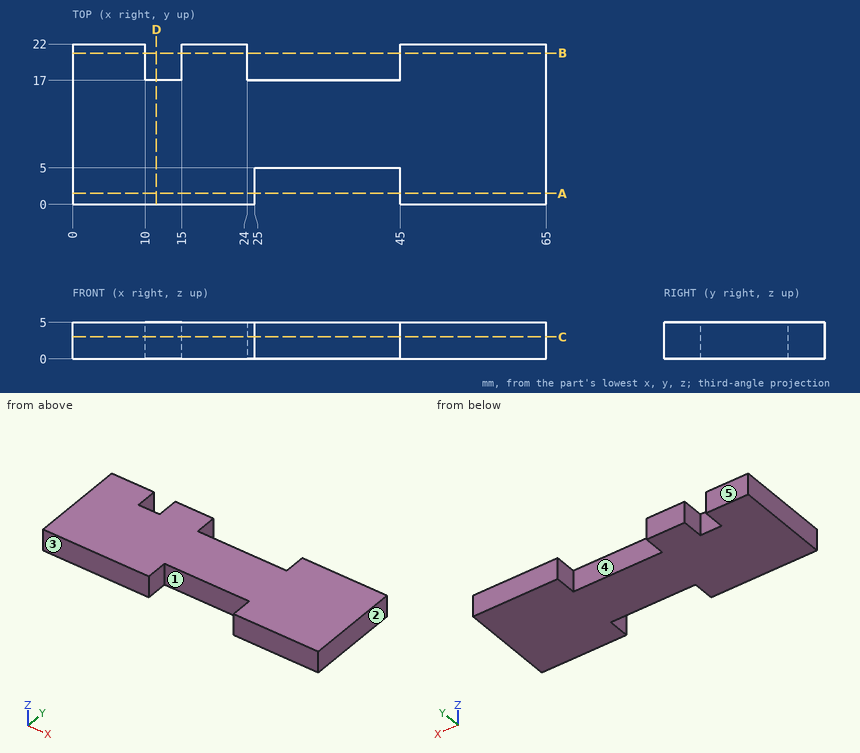
The figure shows three views and two pictorial views of one solid part (mm, origin at its lowest corner). Answer the questions. A direction names the side the tool comes from. Coordinates: 2 decimals unless noted, no trailing zeros. Loops run counter-clockwise (first coordinate to the right, second up) from the corner with the lowest first, then second, coordinate; pieces in that order, holes last. Notation, with made-up numbers: (-30.75, 36.25) -> (3.25, 36.25) arc R22 cw to (3.25, 59.25) -> close; hole circle Ø10 at (-1.75, -9). An arc over 180 degrees is marked (long way). Write item = value, one per line. Start each with the question number.
1) The mould has two halves that part along X. Classify the marked faces 1, 2 and 3: released by +X, released by -X, zero draft, split by the parting line, or undercut.
2) Given pin 1 Ø2.5 at (x, z) = (32.5, 2.5) entering from -Y, flat-ended and moving along its own axis, determine where the tip first touches the part or whether it passes through.
3) A cutting plane is placed at D-D (x = 11.5). Give the vertices of the cut face in (y, z), then the cut area to 3 significant figures.
4) A cutting plane is placed at A-A (y = 1.5). Give the vertices of the cut face in (x, z).
5) Straight lines are drawn through the part: line 1 (X direction, y = 20.75, z = 3.15); line 2 (X direction, y = 3.75, z = 4.4); line 3 (Y direction, x = 43, z = 0.8). For each, find the intervals that lie inside material, in ascending order. Write a range as from..to.
6) A cutting plane is placed at C-C (z = 3). Give the vertices of the cut face in (x, y).
7) A tool of negligible diameter and unlimited length cuts with its end or side. For the marked faces 4 and 5, from which of +Z, -Z, +X, -X, +Y, -Y can it reach the whole face along a straight path? Write none if from no direction.
8) A cutting plane is placed at B-B (y = 20.75). Give the vertices of the cut face in (x, z).
Responses:
q1.face_1 = undercut
q1.face_2 = released by +X
q1.face_3 = zero draft
q2.pin_1 = 5
q3.outline = (0, 0) -> (17, 0) -> (17, 5) -> (0, 5) -> close
q3.area = 85.0 mm²
q4.outline = (0, 0) -> (25, 0) -> (25, 5) -> (0, 5) -> close; (45, 0) -> (65, 0) -> (65, 5) -> (45, 5) -> close
q5.line_1 = 0..10, 15..24, 45..65
q5.line_2 = 0..25, 45..65
q5.line_3 = 5..17
q6.outline = (0, 0) -> (25, 0) -> (25, 5) -> (45, 5) -> (45, 0) -> (65, 0) -> (65, 22) -> (45, 22) -> (45, 17) -> (24, 17) -> (24, 22) -> (15, 22) -> (15, 17) -> (10, 17) -> (10, 22) -> (0, 22) -> close
q7.face_4 = +Z, -Z, +Y
q7.face_5 = +Z, -Z, +X, -X, +Y
q8.outline = (0, 0) -> (10, 0) -> (10, 5) -> (0, 5) -> close; (15, 0) -> (24, 0) -> (24, 5) -> (15, 5) -> close; (45, 0) -> (65, 0) -> (65, 5) -> (45, 5) -> close
